Design review of the part built by this model. Coordinates are the model's own, in mm. A direction names the side the tool comes from. Give positions to 0.01 mm unless a question says otherwise; leave off trailing zeros. Write each loop counter-clockwise with the first axis right and the second up, starting at its lowest first coordinate (ties: lowest second). Pieces come first, ordered by that corner, then holes. Notation, with made-up numbers: M 61.25,22 L 112.25,22 A15 ccw 112.25,42 Z; hole C 11.5,89.25 d5. An arc over 180 degrees is marked long. Write each question's results on one line, items separated by ' | '. Start each with the question number.
Autodesk Inventor part; units mm, degrees
ref_plane "YZ Plane" through (0, 0, 0) normal (1, 0, 0) x (0, 1, 0)
ref_plane "XZ Plane" through (0, 0, 0) normal (0, 1, 0) x (-1, 0, 0)
ref_plane "XY Plane" through (0, 0, 0) normal (0, 0, 1) x (1, 0, 0)
sketch "Sketch1" plane through (0, 0, 0) normal (0, 0, 1) x (1, 0, 0)
  line L0 (-11, 14) -> (11, 14)
  line L1 (11, 14) -> (11, -14)
  line L2 (11, -14) -> (-11, -14)
  line L3 (-11, -14) -> (-11, 14)
  line L4 (-11, 14) -> (11, -14) construction
  line L5 (11, 14) -> (-11, -14) construction
  point P0 (0, 0)
  dimension "d0" = 22
  dimension "d1" = 28
extrude "Extrusion1" add sketch "Sketch1" along normal blind 1.6
sketch "Sketch2" plane through (0, 0, 1.6) normal (0, 0, 1) x (1, 0, 0)
  line L0 (-9, -12) -> (9, -12)
  line L1 (9, -12) -> (9, -1)
  line L2 (9, -1) -> (-9, -1)
  line L3 (-9, -1) -> (-9, -12)
  line L4 (-9, -12) -> (9, -1) construction
  line L5 (9, -12) -> (-9, -1) construction
  line L6 (0, 19.6) -> (0, -19.6)
  line L7 (-11, -14) -> (11, -14)
  point P0 (0, 0)
  point P1 (0, -6.5)
  dimension "d4" = 11
  dimension "d5" = 18
  dimension "d6" = 2
hole "Hole1" at (-9, -1, 1.6) at (9, -1, 1.6) at (9, -12, 1.6) at (-9, -12, 1.6) direction (0, 0, -1) diameter 2.6 end through all
sketch "Sketch3" plane through (0, 0, 1.6) normal (0, 0, 1) x (1, 0, 0)
  line L0 (-2.5, -8.7) -> (2.5, -8.7)
  line L1 (2.5, -8.7) -> (2.5, -4.3)
  line L2 (2.5, -4.3) -> (-2.5, -4.3)
  line L3 (-2.5, -4.3) -> (-2.5, -8.7)
  line L4 (-2.5, -8.7) -> (2.5, -4.3) construction
  line L5 (2.5, -8.7) -> (-2.5, -4.3) construction
  circle A0 centre (9, -1) radius 1.3
  point P0 (0, 0)
  point P1 (0, -6.5)
  dimension "d14" = 5
  dimension "d15" = 4.4
  dimension "d16" = 5.5
extrude "Extrusion2" add sketch "Sketch3" along normal blind 1 contours L3 L2 L1 L0
properties part number "AS5047"
Q1. The part is to be moulded in two halves that separate along X. For faces 1 (the flat face through (11, 0, 1)), 2 (the cylindrical face through (9.5, -13.2, 0.8)), 3 (the flat face through (0, 0, 0)), say which applies: pulls with the +X half, pulls with the -X half, needs draft (parallel to the pull), parting line crosses it, or undercut.
Q2. We need section B-B on x = 9. Write out the cut boundary in (y, z).
Q3. Wall thickness on line 1 along Y through (x, z) = (-9, 0.3); line 2 along X through (y, z) = (-12, 0.9); line 3 along Z through (x, y) = (3, -0.5): over which ranges is each line inside the solid? List them lowest first. Write a range as from..to.
Q4. For pin 1 Ø0.5 at (y, z) = (-6.5, 2) entering from +X; pin 2 Ø0.5 at (y, z) = (-6, 2) entering from -X; pin 3 Ø3 at (x, y) = (-9, -1) entering from +Z, all flat-tipped, find the tip position at first contact; note any pin that passes through.
Q5. We need section D-D on x = 1. Write out the cut boundary in (y, z).
Q6. For faces 4 (the cylindrical face through (-10.29, -0.83, 0.79)), 5 (the flat face through (-2.5, -6, 2)), 6 (the flat face through (2.5, -7, 2)), 7 (the flat face through (0, -4.3, 2)), 8 (the flat face through (0, -8.7, 2)), list the 3-axis set-ups (+Z, -Z, +X, -X, +Y, -Y) from which the entire face can be reached by the end or side of a thin tool; tool diameter is ignored.
Q7. We need section C-C on z = 0.55. Write out the cut boundary in (x, y), and give its area (3 significant figures).
Q8. We need section A-A on y = -12. Write out the cut boundary in (x, z).
Answer sheet:
1) face 1: pulls with the +X half | face 2: undercut | face 3: needs draft
2) outline: M -14,0 L -13.3,0 L -13.3,1.6 L -14,1.6 Z; M -10.7,0 L -2.3,0 L -2.3,1.6 L -10.7,1.6 Z; M 0.3,0 L 14,0 L 14,1.6 L 0.3,1.6 Z
3) line 1: -14..-13.3, -10.7..-2.3, 0.3..14 | line 2: -11..-10.3, -7.7..7.7, 10.3..11 | line 3: 0..1.6
4) pin 1: x = 2.5 | pin 2: x = -2.5 | pin 3: z = 1.6
5) outline: M -14,0 L 14,0 L 14,1.6 L -4.3,1.6 L -4.3,2.6 L -8.7,2.6 L -8.7,1.6 L -14,1.6 Z
6) face 4: +Z, -Z | face 5: +Z, -X, +Y, -Y | face 6: +Z, +X, +Y, -Y | face 7: +Z, +X, -X, +Y | face 8: +Z, +X, -X, -Y
7) outline: M -11,-14 L 11,-14 L 11,14 L -11,14 Z; hole C -9,-12 d2.6; hole C -9,-1 d2.6; hole C 9,-12 d2.6; hole C 9,-1 d2.6 | area: 595 mm^2
8) outline: M -11,0 L -10.3,0 L -10.3,1.6 L -11,1.6 Z; M -7.7,0 L 7.7,0 L 7.7,1.6 L -7.7,1.6 Z; M 10.3,0 L 11,0 L 11,1.6 L 10.3,1.6 Z
